```python
from build123d import *

# Parameters (mm, degrees)
F0_R     = 19.12
F0_R_2   = 11.5
F1_DEPTH = 76.2
F2_R     = 19.12
F3_DEPTH = 27.94
F3_TAPER = 45
F5_DEPTH = 3


with BuildPart() as f1:
    # F0 (on Top) → F1 (new body)
    with BuildSketch(Plane.XY):
        Circle(F0_R)
        Circle(F0_R_2, mode=Mode.SUBTRACT)
    extrude(amount=F1_DEPTH)

    # F2 (on face) → F3 (join)
    with BuildSketch(Plane.XY.offset(76.2)):
        Circle(F2_R)
    extrude(amount=F3_DEPTH, taper=F3_TAPER)

    # F4 (on Front) → F5 (join)
    with BuildSketch(Plane.XZ):
        Polygon((36.165818572, 0), (17.3498187214, 27.032000944), (16.6167281568, 0), align=None)
    extrude(amount=F5_DEPTH)


solid = f1.part
```
For this review, take the finished solid that the model builds, in its own axes (mm). A direction names the side the tool comes from. Give positions to 0.01 mm unless a question says otherwise; leave off trailing zeros. Order: outer loops, then holes, each group sorted by start corner. A loop starts at its lowest first (then second) coordinate and runs counter-clockwise, first axis right, second up.
1) Take a section at A-A (z = 67). Give the boundary of the cut face in (x, y), then the cut area to 3 significant figures.
2) For faces 1 (the face through (24, 0, 7)), 2 (the face through (24, -3, 7)), 3 (the face through (10, -6, 0)), list the 3-axis set-ups (+Z, -Z, +X, -X, +Y, -Y) from which the entire face can be reached by the end or side of a thin tool; tool diameter is ignored.
3) Insertion check: pin 1 (2 mm diameter, centred on y = 8.5, z = 57.5, fed in from -X); pin 2 (5 mm diameter, centred on x = 25, z = 14.5, fed in from -Y); pin 3 (5 mm diameter, centred on x = 10, z = 61.5, fed in from -Y). Each pin has a flat end and moves straight along its axis. Give the tip position at first contact, or say it passes through.
4) The part is to be moulded in two halves that separate along X. For faces 4 (the face through (-0.674, 5.133, 90.143)), 5 (the face through (0, 0, 76.2)), 6 (the face through (27.645, -1.479, 12.241)), 7 (the face through (-1.5, 11.4, 37.6)), say which applies: released by +X, released by -X, zero draft, split by the parting line, or undercut.
5) Take a section at B-B (z = 6). Give the boundary of the cut face in (x, y), then the cut area to 3 significant figures.
6) Wall thickness on line 1 (Y direction, x = 0, z = 31.5); line 2 (Y direction, x = 7.5, z = 10); line 3 (X direction, y = 7, z = 40.5): over which ranges is each line inside the solid? List them lowest first.
Derived:
1. outline: circle Ø38.24 at (0, 0); hole circle Ø23 at (0, 0)
1. area: 733 mm2
2. face 1: +Z, -Z, +X, +Y
2. face 2: +Z, -Z, +X, -Y
2. face 3: -Z, +X, -X, +Y, -Y
3. pin 1: stops at x = -17.59
3. pin 2: stops at y = -3
3. pin 3: stops at y = -17.59
4. face 4: split by the parting line
4. face 5: undercut
4. face 6: released by +X
4. face 7: undercut
5. outline: (18.88, -3) - (31.99, -3) - (31.99, 0) - (19.12, 0) arc R19.12 ccw (long way) to start; hole circle Ø23 at (0, 0)
5. area: 772 mm2
6. line 1: y = -19.12 to -11.5, 11.5 to 19.12
6. line 2: y = -17.59 to -8.72, 8.72 to 17.59
6. line 3: x = -17.79 to -9.12, 9.12 to 17.79
